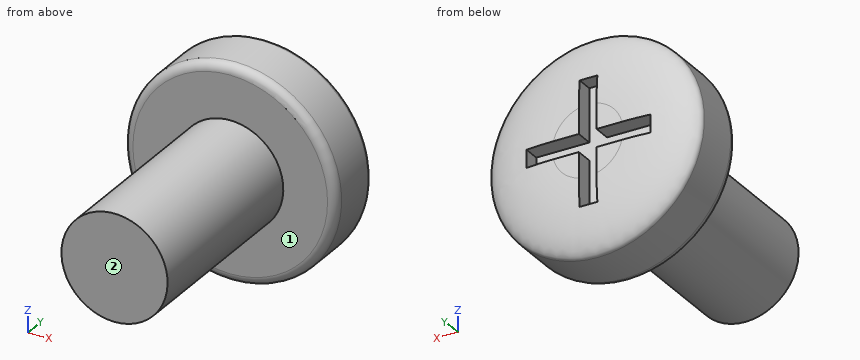
```python
from build123d import *

# Parameters (mm, degrees)
SKETCH1_R           = 3
BOSS_EXTRUDE1_DEPTH = 2
SKETCH2_R           = 1.5
BOSS_EXTRUDE2_DEPTH = 5.5
FILLET2_SIZE        = 0.5
FILLET2_SIZE_2      = 2
SKETCH3_W           = 3.5
SKETCH3_H           = 0.5
SKETCH3_W_2         = 0.5
SKETCH3_H_2         = 3.5
CUT_EXTRUDE1_DEPTH  = 0.5
FILLET3_R           = 0.25


with BuildPart() as part:
    # Sketch1 → Boss-Extrude1 (new body)
    with BuildSketch(Plane(origin=(0, 0, 0), x_dir=(1, 0, 0), z_dir=(0, 1, 0))):
        with Locations(Location((0, 0, 0), (0, 0, 270))):
            Circle(SKETCH1_R)
    extrude(amount=BOSS_EXTRUDE1_DEPTH)

    # Sketch2 → Boss-Extrude2 (add)
    with BuildSketch(Plane.XZ):
        with Locations(Location((0, 0, 0), (0, 0, 270))):
            Circle(SKETCH2_R)
    extrude(amount=BOSS_EXTRUDE2_DEPTH)

    # Fillet2
    # an asymmetric fillet: 2, 0.5 mm, written as the material it takes off along each edge
    with BuildSketch(Plane(origin=(0, 2, 0), x_dir=(0, 0, 1), z_dir=(-1, 0, 0))) as fillet2_piece_1:
        with BuildLine():
            Bezier((3, -FILLET2_SIZE), (3, 0), (3 - FILLET2_SIZE_2, 0), weights=[1, 0.707106781, 1])
            Line((3 - FILLET2_SIZE_2, 0), (3, 0))
            Line((3, 0), (3, -FILLET2_SIZE))
        make_face()
    revolve(axis=Axis((0, 2, 0), (0, 1, 0)), mode=Mode.SUBTRACT)

    # Sketch3 → Cut-Extrude1 (cut)
    with BuildSketch(Plane(origin=(0, 2, 0), x_dir=(1, 0, 0), z_dir=(0, 1, 0))):
        Rectangle(SKETCH3_W, SKETCH3_H)
        Rectangle(SKETCH3_W_2, SKETCH3_H_2)
    extrude(amount=-CUT_EXTRUDE1_DEPTH, mode=Mode.SUBTRACT)

    # Fillet3
    fillet3_edges = [part.edges().sort_by_distance(p)[0] for p in [
        (0, 0, -3),
    ]]
    fillet(fillet3_edges, radius=FILLET3_R)


solid = part.part
```
Build history of the part. All positions in model axes, mm. Face numbers are marked on the shaded views. A direction names the side the tool comes from. Coordinates: 2 decimals unless noted, no trailing zeros. Order: outer loops, then holes, each group sorted by start corner. A loop starts at its lowest first (then second) coordinate and runs counter-clockwise, first axis right, second up.
Item 1: Drop flat-ended pins along their axis: pin 1 Ø1.5 at (x, y) = (0, -3.5) entering from +Z; pin 2 Ø1.5 at (y, z) = (1, -2) entering from +X. Give the stop position or say it passes through.
Filled in:
pin 1: stops at z = 1.5
pin 2: stops at x = 2.73
Item 2: Tool access for the marked faces 1 and 2: list every direction of +Z, -Z, +X, -X, +Y, -Y with a clear straight run to the whole face (end or side of a thin tool).
Filled in:
face 1: -Y
face 2: +Z, -Z, +X, -X, -Y
Item 3: Saw through at B-B on y = 0.5. List the corners of the cut face in (x, z), then the cut area to 3 significant figures.
Filled in:
outline: circle Ø6 at (0, 0)
area: 28.3 mm2
Item 4: Saw through at A-A on y = -3. List the corners of the cut face in (x, z), then the cut area to 3 significant figures.
Filled in:
outline: circle Ø3 at (0, 0)
area: 7.07 mm2
